from build123d import *

# Parameters (mm, degrees)
SKETCH1_W           = 3
SKETCH1_H           = 10
SKETCH1_W_2         = 20
SKETCH1_H_2         = 3
BOSS_EXTRUDE1_DEPTH = 3


with BuildPart() as part:
    # Sketch1 → Boss-Extrude1 (new body)
    with BuildSketch(Plane(origin=(0, 0, 0), x_dir=(1, 0, 0), z_dir=(0, 1, 0))):
        Polygon((0, 0), (0, 10), (-9, 10), (-9, 30), (0, 30), (0, 42.5), (-9, 42.5), (-9, 62.5), (0, 62.5), (0, 75), (-9, 75), (-9, 95), (0, 95), (0, 100), (9.091028316, 95.454485842), (10.432669103, 98.137767415), (19.376941013, 93.66563146), (18.035300226, 90.982349887), (55.601242248, 72.199378876), (56.942883035, 74.882660449), (65.887154945, 70.410524494), (64.545514158, 67.727242921), (102.11145618, 48.94427191), (103.453096967, 51.627553483), (112.397368877, 47.155417528), (111.05572809, 44.472135955), (120, 40), (120, 0), align=None)
        with Locations((116.5, 30)):
            Rectangle(SKETCH1_W, SKETCH1_H, mode=Mode.SUBTRACT)
        with Locations((116.5, 15)):
            Rectangle(SKETCH1_W, SKETCH1_H, mode=Mode.SUBTRACT)
        with Locations((30, 4.5)):
            Rectangle(SKETCH1_W_2, SKETCH1_H_2, mode=Mode.SUBTRACT)
        with Locations((95, 4.5)):
            Rectangle(SKETCH1_W_2, SKETCH1_H_2, mode=Mode.SUBTRACT)
        with Locations((-4.5, 85)):
            Rectangle(SKETCH1_W, SKETCH1_H, mode=Mode.SUBTRACT)
        with Locations((-4.5, 52.5)):
            Rectangle(SKETCH1_W, SKETCH1_H, mode=Mode.SUBTRACT)
        with Locations((-4.5, 20)):
            Rectangle(SKETCH1_W, SKETCH1_H, mode=Mode.SUBTRACT)
    extrude(amount=BOSS_EXTRUDE1_DEPTH)


solid = part.part
Part model, mm, in its own coordinate system. A direction names the side the tool comes from. Coordinates: 2 decimals unless noted, no trailing zeros. Write each loop counter-clockwise with the first axis right and the second up, starting at its lowest first coordinate (ties: lowest second). Pieces come first, ordered by that corner, then holes. Notation, with made-up numbers: M 15,21 L 55,21 A12 cw 55,31 Z; hole C 24,-3.75 d7. An arc over 180 degrees is marked long. Return JSON: item names as keys, results as strings.
1. Saw through at C-C, the plane y = 1.8. Count the separate pieces of the cut face and the enclosed holes in it, then the cut area to 3 significant figures.
Determined:
{"separate pieces": "1", "enclosed holes": "7", "area": "8,760 mm²"}
2. Pull direction Z, two halves, no side cores. Call faces 4 (the face through (-9, 1, -85)), 5 (the face through (111.736, 1.479, -45.833)), 6 (the face through (116, 1, -35)), 7 (the face through (61, 1, 0)): pulls with the +Z half, pulls with the -Z half, needs draft (parallel to the pull), parting line crosses it, or undercut.
Determined:
{"face 4": "needs draft", "face 5": "undercut", "face 6": "undercut", "face 7": "pulls with the +Z half"}
3. Flat gauge pins, fed straight in: pin 1 Ø0.9 at (x, y) = (-4, 2) entering from +Z; pin 2 Ø1.5 at (y, z) = (1.5, -5.5) entering from -X; pin 3 Ø0.9 at (y, z) = (1.5, -51) entering from +X. Where does each tip first touch, or does it go through?
Determined:
{"pin 1": "z = -10", "pin 2": "x = 0", "pin 3": "x = 105.61"}
4. Saw through at A-A, the plane x = 34. Write the cut outline in (y, z), then the cut area to 3 significant figures.
Determined:
{"outline": "M 0,-83 L 3,-83 L 3,-6 L 0,-6 Z; M 0,-3 L 3,-3 L 3,0 L 0,0 Z", "area": "240 mm²"}
5. Saw through at B-B, the plane z = -22. Write the cut outline in (x, y).
Determined:
{"outline": "M -9,0 L -6,0 L -6,3 L -9,3 Z; M -3,0 L 120,0 L 120,3 L -3,3 Z"}
6. Probe L1, parallel to Z at x = 115.5, y = 2.1; L2, parallel to X at y = 0.5, z = -11.5; L3, parallel to Z at x = 112, y = 1.45. List the from-to ranges inside material, lowest first.
Determined:
{"L1": "-42.25 to -35, -25 to -20, -10 to 0", "L2": "-9 to 115, 118 to 120", "L3": "-47.35 to -46.36, -44 to 0"}
7. 3-axis set-ups, long thin cutter, end or side, ignore diameter. For faces 1 (the face through (30, 1, -3)), 2 (the face through (56.26, 1.48, -73.52)), 3 (the face through (-5, 1, -30)): which of +Z, -Z, +X, -X, +Y, -Y reach the whole face in a straight line?
Determined:
{"face 1": "+Y, -Y", "face 2": "-Z, +Y, -Y", "face 3": "-X, +Y, -Y"}
8. Saw through at D-D, the plane x = 73. Write the cut outline in (y, z), then the cut area to 4 significant figures.
Determined:
{"outline": "M 0,-63.5 L 3,-63.5 L 3,0 L 0,0 Z", "area": "190.5 mm²"}
